Model file for the job. Use its own axes, mm. Face numbers are marked on the shaded views. A direction names the side the tool comes from. Round coordinates to 2 decimals unless told otherwise and drop trailing zeros. Loops run counter-clockwise (first coordinate to the right, second up) from the corner with the lowest first, then second, coordinate; pieces in that order, holes last. Notation, with made-up numbers: M 89,47.25 L 112,47.25 A29 ccw 112,69.25 Z; hole C 75,-5.75 d2. An arc over 180 degrees is marked long. Use a Markdown table: item, result. Add a question column.
Q1. Mould opens along Y. For the marked faces 6, 7 and 8 say: +Y half, -Y half, draft (parallel to the pull), parting line (faces both ways), or undercut.
Q2. Probe line 1 (Z direction, x = -3, y = -4) (3 decimals); line 2 (X direction, y = -3.25, z = -2.5); line 3 (X direction, y = -1, z = -4.25). List the from-to ranges inside material, lowest first. Write a range as from..to.
Q3. Cut at B-B (y = -0.5). Give the cut face in (x, z).
Q4. Pin check, flat tips, straight feed: pin 1 (1 mm diameter, centred on y = 3.5, z = 5, fed in from +X); pin 2 (4 mm diameter, centred on x = 0, y = -2, fed in from -Z); pin 3 (5 mm diameter, centred on y = -4, z = -5.5, fed in from -X); pin 4 (6.5 mm diameter, centred on y = -1.5, z = -0.5, fed in from +X). Stop position of each tip, or through.
Q5. Cut at A-A (x = 0). State how many separate pieces and enclosed holes the cut face has, plus the area to 3 significant figures.
Q6. Tool access for the marked faces 1, 2, 3, 4 and 5: list every direction of +Z, -Z, +X, -X, +Y, -Y with a clear straight run to the whole face (end or side of a thin tool).
from build123d import *

# Parameters (mm, degrees)
SKETCH1_R                     = 7.5
BOSS_EXTRUDE1_DEPTH           = 19
BOSS_EXTRUDE1_TAPER           = 2
BOSS_EXTRUDE1_OTHER_WAY_DEPTH = 6
BOSS_EXTRUDE1_OTHER_WAY_TAPER = -2
CUT_EXTRUDE1_DEPTH            = 22.90601606
CUT_EXTRUDE1_DEPTH_BACK       = 22.90601606
CUT_EXTRUDE2_START            = -9.595582485
CUT_EXTRUDE2_OUTLINE_W        = 6.502745185
CUT_EXTRUDE2_OUTLINE_H        = 6
CUT_EXTRUDE2_DEPTH            = 9.595582485
SKETCH5_R                     = 1.5
CUT_EXTRUDE3_DEPTH            = 25.014303442
FILLET1_SIZE                  = 5
CUT_EXTRUDE4_DEPTH            = 22.833157665
CUT_EXTRUDE4_DEPTH_BACK       = 22.833157665
SKETCH6_W                     = 18.67842866
SKETCH6_H                     = 10.820279471
CUT_EXTRUDE5_DEPTH            = 19.604050317


with BuildPart() as part:
    # Sketch1 → Boss-Extrude1 (new body)
    with BuildSketch(Plane(origin=(0, 0, 0), x_dir=(1, 0, 0), z_dir=(0, 1, 0))):
        Circle(SKETCH1_R)
    extrude(amount=BOSS_EXTRUDE1_DEPTH, taper=BOSS_EXTRUDE1_TAPER)

    # Sketch1 → Boss-Extrude1 other way (add)
    with BuildSketch(Plane(origin=(0, 0, 0), x_dir=(1, 0, 0), z_dir=(0, 1, 0))):
        Circle(SKETCH1_R)
    extrude(amount=-BOSS_EXTRUDE1_OTHER_WAY_DEPTH, taper=BOSS_EXTRUDE1_OTHER_WAY_TAPER)

    # Sketch3 → Cut-Extrude1 (cut, two sides: drawn at the far end of the back side and taken through both)
    with BuildSketch(Plane(origin=(0, 0, 0), x_dir=(0, 0, -1), z_dir=(1, 0, 0)).offset(-CUT_EXTRUDE1_DEPTH_BACK)):
        Polygon((-1.886057768, -6), (-1.886057768, 0), (-9.929766736, 8.043708969), (-9.929766736, -6), align=None)
    extrude(amount=CUT_EXTRUDE1_DEPTH + CUT_EXTRUDE1_DEPTH_BACK, mode=Mode.SUBTRACT)

    # Cut-Extrude2: read off the stored shape, not the designer's step
    # Cut-Extrude2 outline → Cut-Extrude2 (cut)
    with BuildSketch(Plane.XY.offset(1.886057768).offset(CUT_EXTRUDE2_START)):
        with Locations((-8.251372593, -3)):
            Rectangle(CUT_EXTRUDE2_OUTLINE_W, CUT_EXTRUDE2_OUTLINE_H)
        with Locations((8.251372593, -3)):
            Rectangle(CUT_EXTRUDE2_OUTLINE_W, CUT_EXTRUDE2_OUTLINE_H)
    extrude(amount=CUT_EXTRUDE2_DEPTH, mode=Mode.SUBTRACT)

    # Sketch5 → Cut-Extrude3 (cut, through all)
    with BuildSketch(Plane(origin=(5, 0, 0), x_dir=(0, 0, -1), z_dir=(1, 0, 0))):
        with Locations((0.613942232, -3.5)):
            Circle(SKETCH5_R)
    extrude(amount=-CUT_EXTRUDE3_DEPTH, mode=Mode.SUBTRACT)

    # Fillet1
    # a fillet whose section is not a circle: 5 mm, written as the material it takes off along each edge
    with BuildSketch(Plane(origin=(17.5, -6, 1.886057768), x_dir=(0, 0, -1), z_dir=(-1, 0, 0))) as fillet1_piece_1:
        with BuildLine():
            Bezier((FILLET1_SIZE, 0), (0, 0), (0, -FILLET1_SIZE), weights=[1, 1.5, 1])
            Line((0, -FILLET1_SIZE), (0, 0))
            Line((0, 0), (FILLET1_SIZE, 0))
        make_face()
    extrude(amount=35, mode=Mode.SUBTRACT)

    # Fillet2
    # a fillet whose section is not a circle: 10, 5 mm, written as the material it takes off along each edge
    with BuildSketch(Plane(origin=(0, 19, 0), x_dir=(1, 0, 0), z_dir=(0, 0, -1))) as fillet2_piece_1:
        with BuildLine():
            Bezier((7.179619488, 9.825502516), (6.83650538, 0), (2.182665353, 0), weights=[1, 0.818181818, 1])
            Line((2.182665353, 0), (6.83650538, 0))
            Line((6.83650538, 0), (7.179619488, 9.825502516))
        make_face()
    revolve(axis=Axis((0, 19, 0), (0, -1, 0)), mode=Mode.SUBTRACT)

    # Sketch6 → Cut-Extrude4 (cut, two sides: drawn at the far end of the back side and taken through both)
    with BuildSketch(Plane(origin=(0, 0, 0), x_dir=(0, 0, -1), z_dir=(1, 0, 0)).offset(-CUT_EXTRUDE4_DEPTH_BACK)):
        with Locations((-1.153671222, 14.589860265)):
            Rectangle(SKETCH6_W, SKETCH6_H)
    extrude(amount=CUT_EXTRUDE4_DEPTH + CUT_EXTRUDE4_DEPTH_BACK, mode=Mode.SUBTRACT)

    # Sketch7 → Cut-Extrude5 (cut, through all)
    with BuildSketch(Plane.XZ.offset(6)):
        with BuildLine():
            Line((4, -3.113942232), (4, -4.074146702))
            ThreePointArc((4, -4.074146702), (0, -5.709524617), (-4, -4.074146702))
            Line((-4, -4.074146702), (-4, -3.113942232))
            Line((-4, -3.113942232), (4, -3.113942232))
        make_face()
    extrude(amount=-CUT_EXTRUDE5_DEPTH, mode=Mode.SUBTRACT)


solid = part.part
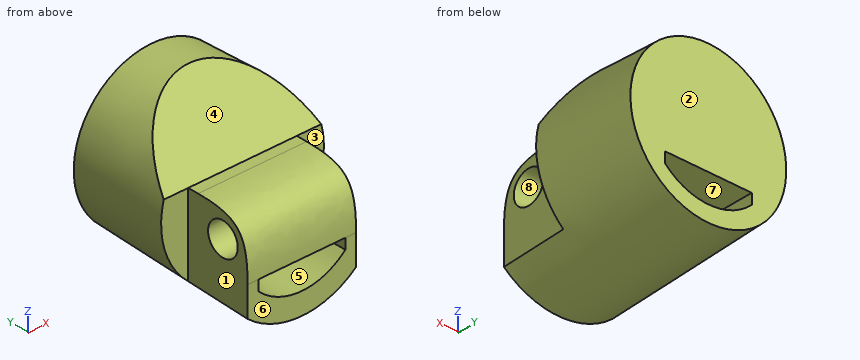
Checked values:
| question | item | result |
|---|---|---|
| 1 | face 6 | -Y half |
| 1 | face 7 | draft |
| 1 | face 8 | undercut |
| 2 | line 1 | z = -7.026..-4.858, -3.114..-2.028, 0.8..1.505 |
| 2 | line 2 | x = -5..5 |
| 2 | line 3 | x = -5..-3.81, 3.81..5 |
| 3 | outline | M -5,-5.61 A7.52 ccw 5,-5.61 L 5,1.89 L -5,1.89 Z; hole M -4,-4.07 A5.71 ccw 4,-4.07 L 4,-3.11 L -4,-3.11 Z |
| 4 | pin 1 | stops at x = 5.85 |
| 4 | pin 2 | stops at z = -7.64 |
| 4 | pin 3 | stops at x = -5 |
| 4 | pin 4 | stops at x = 7.5 |
| 5 | separate pieces | 2 |
| 5 | enclosed holes | 1 |
| 5 | area | 127 mm^2 |
| 6 | face 1 | +Z, -Z, -X, -Y |
| 6 | face 2 | +Z, -Z, +X, -X, +Y |
| 6 | face 3 | +Z, -Z, +X, -Y |
| 6 | face 4 | +Z, +X, -X, -Y |
| 6 | face 5 | +Y, -Y |
